Autodesk Inventor part; units mm, degrees
ref_plane "YZ Plane" through (0, 0, 0) normal (1, 0, 0) x (0, 1, 0)
ref_plane "XZ Plane" through (0, 0, 0) normal (0, 1, 0) x (-1, 0, 0)
ref_plane "XY Plane" through (0, 0, 0) normal (0, 0, 1) x (1, 0, 0)
sketch "Sketch1" plane through (0, 0, 0) normal (0, 1, 0) x (-1, 0, 0)
  line L0 (-40, -47.5) -> (40, -47.5)
  line L1 (40, -47.5) -> (40, 47.5)
  line L2 (40, 47.5) -> (-40, 47.5)
  line L3 (-40, 47.5) -> (-40, -47.5)
  line L4 (-40, -47.5) -> (40, 47.5) construction
  line L5 (40, -47.5) -> (-40, 47.5) construction
  line L6 (25.5, 17) -> (28.5, 17)
  line L7 (0, 17.5) -> (0, 19)
  line L8 (0, 0) -> (2.25, 0)
  line L9 (0, 0) -> (0, 17.5)
  line L10 (-27.5, -36.75) -> (-27.5, 38.25)
  line L11 (-27.5, 38.25) -> (28.5, -36.75) construction
  line L12 (28.5, 38.25) -> (-27.5, -36.75) construction
  line L13 (28.5, 38.25) -> (28.5, -36.75)
  line L14 (28.5, 17) -> (28.5, -36.75)
  line L15 (28.5, -36.75) -> (-27.5, -36.75)
  line L16 (0, -31.5) -> (8.5, -31.5)
  line L17 (0, 0) -> (0, -31.5)
  line L18 (0, -31.5) -> (-19.5, -31.5)
  line L19 (-19.5, -31.5) -> (-19.5, -36.75)
  line L20 (-27.5, 38.25) -> (28.5, 38.25)
  line L21 (0, 19) -> (24, 19)
  line L22 (0, 0) -> (0, 31.5)
  line L23 (28.5, -17) -> (28.5, 36.75)
  line L24 (28.5, -38.25) -> (28.5, 36.75)
  line L25 (28.5, -38.25) -> (-27.5, 36.75) construction
  line L26 (-27.5, 36.75) -> (-27.5, -38.25)
  line L27 (-27.5, -38.25) -> (28.5, 36.75) construction
  line L28 (0, 31.5) -> (8.5, 31.5)
  circle A0 centre (8.5, 31.5) radius 2.5
  line L29 (0, 31.5) -> (-19.5, 31.5)
  circle A1 centre (-19.5, 31.5) radius 2.5
  circle A2 centre (-19.5, 31.5) radius 2.5
  line L30 (-19.5, 31.5) -> (-19.5, 36.75)
  line L31 (28.5, 36.75) -> (-27.5, 36.75)
  line L32 (0, 0) -> (0, -17.5)
  line L33 (0, -17.5) -> (0, -19)
  line L34 (25.5, -17) -> (28.5, -17)
  line L35 (0, -19) -> (24, -19)
  line L36 (-27.5, -38.25) -> (28.5, -38.25)
  circle A3 centre (24, -19) radius 2.5
  point P0 (0.5, 0.75)
  point P1 (0.5, -0.75)
  dimension "d0" = 80
  dimension "d1" = 95
  dimension "d5" = 17.5
  dimension "d6" = 8.5
  dimension "d7" = 19.5
  dimension "d8" = 31.5
  dimension "d9" = 24
  dimension "d11" = 2.25
  dimension "d12" = 56
  dimension "d13" = 75
  dimension "d14" = 5.25
  dimension "d15" = 3
ref_plane "Work Plane3" through (0, 10, 0) normal (0, 1, 0) x (1, 0, 0)
sketch "Sketch2" plane through (0, 10, 0) normal (0, 1, 0) x (1, 0, 0)
  line L0 (35.5, -47.5) -> (40, -39.7058)
  line L1 (35.5, -47.5) -> (44.5, -47.5) construction
  line L2 (40, -39.7058) -> (35.5, -39.7058)
  line L3 (35.5, -39.7058) -> (35.5, -47.5)
  line L4 (-40, -47.5) -> (40, -47.5)
  line L5 (40, -47.5) -> (40, 47.5)
  line L6 (40, -37.7058) -> (33.5, -37.7058)
  line L7 (33.5, -37.7058) -> (33.5, -47.5)
  line L8 (33.5, -47.5) -> (35.5, -47.5)
  line L9 (40, -39.7058) -> (40, -37.7058)
  line L10 (0, -47.5) -> (0, 47.5)
  line L11 (-35.5, -47.5) -> (-40, -39.7058)
  line L12 (-35.5, -47.5) -> (-44.5, -47.5) construction
  line L13 (-40, -39.7058) -> (-35.5, -39.7058)
  line L14 (-35.5, -39.7058) -> (-35.5, -47.5)
  line L15 (-40, -37.7058) -> (-33.5, -37.7058)
  line L16 (-33.5, -37.7058) -> (-33.5, -47.5)
  line L17 (-33.5, -47.5) -> (-35.5, -47.5)
  line L18 (-40, -39.7058) -> (-40, -37.7058)
  line L19 (40, 47.5) -> (-40, 47.5)
  line L20 (-40, 47.5) -> (-33.5, 47.5)
  line L21 (-33.5, 47.5) -> (-33.5, 37.5)
  line L22 (-33.5, 37.5) -> (-40, 37.5)
  line L23 (-40, 37.5) -> (-40, 47.5)
  line L24 (40, 47.5) -> (33.5, 47.5)
  line L25 (33.5, 47.5) -> (33.5, 37.5)
  line L26 (33.5, 37.5) -> (40, 37.5)
  line L27 (40, 37.5) -> (40, 47.5)
  point P0 (0, 0)
  dimension "d18" = 9
  dimension "d19" = 60
  dimension "d20" = 2
  dimension "d21" = 9.7942
  dimension "d22" = 6.5
  dimension "d23" = 6.5
  dimension "d24" = 10
  dimension "d25" = 6.5
  dimension "d26" = 10
extrude "Extrusion2" add sketch "Sketch2" along normal blind 100 contours L3 L2 L0 | L4 L7 L6 L5 L2 L3 | L26 L25 L19 L5 | L14 L13 L18 L15 L16 L4 | L11 L13 L14 | L21 L22 L23 L19
ref_plane "Work Plane2" through (0, 10, 0) normal (0, 1, 0) x (1, 0, 0)
sketch "Sketch3" plane through (0, 10, 0) normal (0, 1, 0) x (1, 0, 0)
  line L0 (-40, 37.5) -> (-40, -37.7058)
  line L1 (-33.5, 37.5) -> (-40, 37.5)
  line L2 (-40, -37.7058) -> (-36.75, -37.7058)
  line L3 (-36.75, -37.7058) -> (-36.75, 37.5)
  line L4 (-36.75, 37.5) -> (-40, 37.5)
  line L5 (-40, 37.5) -> (-40, -37.7058)
  line L6 (33.5, 37.5) -> (40, 37.5)
  line L7 (40, -37.7058) -> (33.5, -37.7058)
  line L8 (40, 37.5) -> (36.75, 37.5)
  line L9 (36.75, 37.5) -> (36.75, -37.7058)
  line L10 (36.75, -37.7058) -> (40, -37.7058)
  line L11 (40, -37.7058) -> (40, 37.5)
  point P0 (0, 0)
extrude "Extrusion3" add sketch "Sketch3" along normal blind 5
ref_plane "Work Plane4" through (0, 110, 0) normal (0, 1, 0) x (1, 0, 0)
sketch "Sketch4" plane through (0, 110, 0) normal (0, 1, 0) x (1, 0, 0)
  line L0 (-33.5, 47.5) -> (-40, 47.5)
  line L1 (-40, -47.5) -> (40, -47.5)
  line L2 (-40, 47.5) -> (-33.5, 47.5)
  line L3 (-33.5, 47.5) -> (-33.5, -47.5)
  line L4 (-33.5, -47.5) -> (-40, -47.5)
  line L5 (-40, -47.5) -> (-40, 47.5)
  line L6 (40, 37.5) -> (40, 47.5)
  line L7 (40, 47.5) -> (33.5, 47.5)
  line L8 (33.5, 47.5) -> (33.5, -47.5)
  line L9 (33.5, -47.5) -> (40, -47.5)
  line L10 (40, -47.5) -> (40, 47.5)
  line L11 (40, -37.7058) -> (33.5, -37.7058)
  line L12 (33.5, -37.7058) -> (-33.5, -37.7058)
  line L13 (-33.5, -37.7058) -> (-33.5, -47.5)
  line L14 (-33.5, -47.5) -> (33.5, -47.5)
  line L15 (33.5, -47.5) -> (33.5, -37.7058)
  point P0 (0, 0)
extrude "Extrusion4" add sketch "Sketch4" along normal blind 8
ref_plane "Work Plane8" through (40, 0, -47.5) normal (0, 0, -1) x (-1, 0, 0)
sketch "Sketch5" plane through (40, 0, -47.5) normal (0, 0, -1) x (-1, 0, 0)
  line L0 (73.5, 110) -> (6.5, 110)
  line L1 (6.5, 110) -> (6.5, 113)
  line L2 (6.5, 10) -> (6.5, 118)
  line L3 (6.5, 113) -> (3.25, 113)
  line L4 (3.25, 113) -> (3.25, 116)
  line L5 (3.25, 116) -> (6.5, 116)
  line L6 (6.5, 116) -> (6.5, 113)
  line L7 (73.5, 10) -> (73.5, 118)
  line L8 (6.5, 116) -> (73.5, 116)
  line L9 (73.5, 116) -> (73.5, 113)
  line L10 (73.5, 113) -> (6.5, 113)
  line L11 (6.5, 113) -> (6.5, 116)
  line L12 (73.5, 113) -> (76.75, 113)
  line L13 (76.75, 113) -> (76.75, 116)
  line L14 (76.75, 116) -> (73.5, 116)
  line L15 (73.5, 116) -> (73.5, 113)
  point P0 (40, 0)
  dimension "d33" = 3
  dimension "d34" = 3
  dimension "d35" = 3.25
  dimension "d36" = 3.25
extrude "Extrusion5" cut sketch "Sketch5" against normal blind 90.206 contours L10 L2 L8 L7 | L7 L14 L13 L12 | L3 L4 L5 L2
ref_plane "Work Plane7" through (40, 10, 39.7058) normal (0.8660254, 0, 0.5) x (0.5, 0, -0.8660254)
sketch "Sketch6" plane through (40, 10, 39.7058) normal (0.8660254, 0, 0.5) x (0.5, 0, -0.8660254)
  line L0 (-9, 0) -> (-9, 100)
  line L1 (0, 0) -> (-9, 0)
  line L2 (-9, 100) -> (0, 100)
  line L3 (0, 100) -> (0, 0)
  line L4 (0, 0) -> (-9, 0)
  line L5 (-9, 0) -> (-9, 100)
  line L6 (0, 100) -> (0, 70)
  line L7 (0, 0) -> (0, 100)
  line L8 (0, 70) -> (-4.5, 70)
  circle A0 centre (-4.5, 70) radius 1.5
  point P0 (14.3862, -10)
  dimension "d39" = 30
  dimension "d40" = 3
extrude "Extrusion6" cut sketch "Sketch6" against normal blind 6 contours A0
ref_plane "Work Plane6" through (-35.5, 10, 47.5) normal (-0.8660254, 0, 0.5) x (0.5, 0, 0.8660254)
sketch "Sketch7" plane through (-35.5, 10, 47.5) normal (-0.8660254, 0, 0.5) x (0.5, 0, 0.8660254)
  line L0 (-9, 0) -> (-9, 100)
  line L1 (0, 0) -> (0, 100)
  line L2 (-9, 100) -> (0, 100)
  line L3 (0, 100) -> (0, 0)
  line L4 (0, 0) -> (-9, 0)
  line L5 (-9, 0) -> (-9, 100)
  line L6 (-9, 100) -> (-9, 70)
  line L7 (-9, 70) -> (-4.5, 70)
  circle A0 centre (-4.5, 70) radius 1.5
  point P0 (-23.3862, -10)
  dimension "d43" = 30
  dimension "d44" = 3
extrude "Extrusion7" cut sketch "Sketch7" against normal blind 6 contours A0
ref_plane "Work Plane5" through (40, 0, 47.5) normal (1, 0, 0) x (0, 0, -1)
sketch "Sketch8" plane through (40, 0, 47.5) normal (1, 0, 0) x (0, 0, -1)
  line L0 (85, 110) -> (9.7942, 110)
  line L1 (85, 110) -> (95, 110)
  line L2 (95, 110) -> (95, 80)
  line L3 (95, 80) -> (85, 80)
  line L4 (85, 80) -> (85, 110)
  circle A0 centre (90, 80) radius 1.5
  point P0 (47.5, 0)
  dimension "d47" = 10
  dimension "d48" = 30
  dimension "d49" = 3
extrude "Extrusion8" [suppressed]
ref_plane "Work Plane1" through (0, 0, 0) normal (0, -1, 0) x (1, 0, 0)
sketch "Sketch9" plane through (0, 0, 0) normal (0, -1, 0) x (1, 0, 0)
  line L0 (40, 47.5) -> (40, 39.7058)
  line L1 (40, 47.5) -> (20, 47.5)
  line L2 (20, 47.5) -> (20, -10)
  line L3 (20, -10) -> (40, -10)
  line L4 (40, -10) -> (40, 47.5)
  line L5 (-40, 47.5) -> (-35.5, 47.5)
  line L6 (-40, 47.5) -> (-20, 47.5)
  line L7 (-20, 47.5) -> (-20, -10)
  line L8 (-20, -10) -> (-40, -10)
  line L9 (-40, -10) -> (-40, 47.5)
  point P0 (0, 0)
  dimension "d52" = 20
  dimension "d53" = 57.5
  dimension "d54" = 20
  dimension "d55" = 57.5
extrude "Extrusion9" add sketch "Sketch1" along normal blind 10 contours L3 L2 L1 L0 | L9 L17 L18 L19 L15 L10 L31 L30 A1 L29 L22 L7 | L7 L22 L29 A1 L30 L31 L13 L34 A3 L35 L17 L9 | L35 A3 L34 L13 L15 L19 L18 L17 | L31 L10 L20 L13 | L15 L24 L36 L26
properties part number "Base"
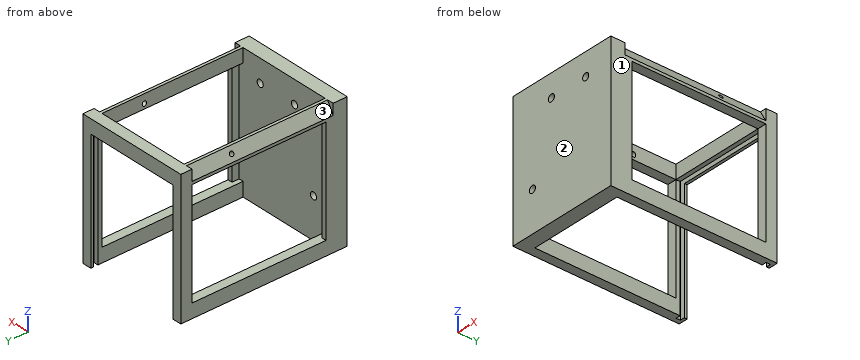
Model file for the job. Use its own axes, mm. Face numbers are marked on the shaded views. Coordinates: 2 decimals unless noted, no trailing zeros. Write each loop counter-clockwise with the first axis right and the second up, starting at its lowest first coordinate (ties: lowest second). Pieces come first, ordered by that corner, then holes. Notation, with made-up numbers: (2.25, 24) - (34.25, 24) arc R25 cw to (34.25, 59) - close; hole circle Ø9 at (-21, 38). An arc over 180 degrees is marked (long way). Write each question's results on one line, items separated by ' | '. Start each with the question number.
1) Probe line 1 along X through (y, z) = (6.25, 31.5); line 2 along Y through (x, z) = (35.5, -20); line 3 along Z through (x, y) = (-24, 6.5). List the from-to ranges inside material, lowest first. Write a range as from..to.
2) Cut at D-D (x = 7.5). Write the cut outline in (y, z), then the cut area to 3 significant figures.
3) Cut at B-B (x = -24). Write the cut outline in (y, z), then the cut area to 3 significant figures.
4) Mould opens along Y. For the marked faces 1, 2 and 3 say: pulls with the +Y half, pulls with the -Y half, needs draft (parallel to the pull), parting line crosses it, or undercut.
5) Cut at C-C (z = -19). Write the cut outline in (x, y), then the cut area to 3 significant figures.
6) Flat gauge pins, fed straight in: P1, Ø3, axis at x = -19.5, z = 12, coming from the +Y side; P2, Ø3.5, axis at x = -11.5, y = 114, coming from the -Z side. Where does each tip first touch, or does it go through?
7) Cut at A-A (z = 21). Write the cut outline in (x, y), then the cut area to 3 significant figures.
Returned:
1) line 1: -40..-11, -6..17, 22..40 | line 2: 0..10, 110..113, 116..118 | line 3: -47.5..-21.5, -16.5..47.5
2) outline: (0, -47.5) - (10, -47.5) - (10, 47.5) - (0, 47.5) - close; (110, 37.71) - (113, 37.71) - (113, 42.71) - (116, 42.71) - (116, 37.71) - (118, 37.71) - (118, 47.5) - (110, 47.5) - close | area: 1,010 mm^2
3) outline: (0, -47.5) - (10, -47.5) - (10, -21.5) - (0, -21.5) - close; (0, -16.5) - (10, -16.5) - (10, 47.5) - (0, 47.5) - close; (110, 37.71) - (113, 37.71) - (113, 42.71) - (116, 42.71) - (116, 37.71) - (118, 37.71) - (118, 47.5) - (110, 47.5) - close | area: 963 mm^2
4) face 1: needs draft | face 2: pulls with the -Y half | face 3: undercut
5) outline: (-40, 0) - (-26.5, 0) - (-26.5, 10) - (-36.75, 10) - (-36.75, 15) - (-40, 15) - close; (-40, 110) - (-33.5, 110) - (-33.5, 113) - (-36.75, 113) - (-36.75, 116) - (-33.5, 116) - (-33.5, 118) - (-40, 118) - close; (-21.5, 0) - (40, 0) - (40, 15) - (36.75, 15) - (36.75, 10) - (-21.5, 10) - close; (33.5, 110) - (40, 110) - (40, 118) - (33.5, 118) - (33.5, 116) - (36.75, 116) - (36.75, 113) - (33.5, 113) - close | area: 867 mm^2
6) P1: y = 10 | P2: z = 37.71
7) outline: (-40, 0) - (40, 0) - (40, 15) - (36.75, 15) - (36.75, 10) - (-36.75, 10) - (-36.75, 15) - (-40, 15) - close; (-40, 110) - (-33.5, 110) - (-33.5, 113) - (-36.75, 113) - (-36.75, 116) - (-33.5, 116) - (-33.5, 118) - (-40, 118) - close; (33.5, 110) - (40, 110) - (40, 118) - (33.5, 118) - (33.5, 116) - (36.75, 116) - (36.75, 113) - (33.5, 113) - close | area: 917 mm^2
